Autodesk Inventor part; units mm, degrees
ref_plane "Work Plane1" through (-5.75, 2, 0) normal (0, 1, 0) x (1, 0, 0)
ref_plane "YZ Plane" through (0, 0, 0) normal (1, 0, 0) x (0, 1, 0)
ref_plane "XZ Plane" through (0, 0, 0) normal (0, 1, 0) x (-1, 0, 0)
sketch "Sketch1" plane through (0, 0, 0) normal (0, 0, 1) x (1, 0, 0)
  circle A0 centre (0, 0) radius 1
  circle A1 centre (0, 0) radius 1.75
  line L0 (-1.75, 0) -> (-1.75, -4)
  line L1 (-1.75, -4) -> (-5.75, -4)
  line L2 (-5.75, -4) -> (-5.75, -6)
  line L3 (-5.75, -6) -> (0, -6)
  line L4 (0, 0) -> (0, -6)
  line L5 (1.75, 0) -> (1.75, -4)
  line L6 (1.75, -4) -> (5.75, -4)
  line L7 (5.75, -4) -> (5.75, -6)
  line L8 (5.75, -6) -> (0, -6)
  dimension "d9" = 3.5
  dimension "d8" = 2
  dimension "d10" = 4
  dimension "d11" = 4
  dimension "d12" = 2
  dimension "d13" = 5.75
extrude "Extrusion1" add sketch "Sketch1" along normal blind 12
ref_plane "Work Plane1" through (-5.75, 2, 0) normal (0, 1, 0) x (1, 0, 0)
sketch "Sketch2" plane through (-5.75, 2, 0) normal (0, 1, 0) x (1, 0, 0)
  line L0 (7.5, 0) -> (7.5, -12)
  line L1 (4, 0) -> (7.5, 0)
  line L2 (4, 0) -> (4, -12)
  line L3 (4, -12) -> (7.5, -12)
  line L4 (6.75, -12) -> (4.75, -12) construction
  line L5 (5.75, -12) -> (5.75, 0) construction
  line L6 (7.5, -6) -> (4, -6) construction
  line L7 (4, 0) -> (4, -12) construction
  line L8 (7.5, -10.5) -> (4, -10.5)
  line L9 (4, -10.5) -> (4, -1.5)
  line L10 (4, -1.5) -> (7.5, -1.5)
  line L11 (7.5, -1.5) -> (7.5, -10.5)
  line L12 (7.5, -10.5) -> (4, -1.5) construction
  line L13 (4, -10.5) -> (7.5, -1.5) construction
  point P0 (5.75, -6)
  dimension "d17" = 9
extrude "Extrusion2" cut sketch "Sketch2" against normal blind 12 contours L0 L8 L2 L10
fillet "Fillet1" radius 2 4 edges at (1.75, -4, 0.75) (1.75, -4, 11.25) (-1.75, -4, 0.75) (-1.75, -4, 11.25)
fillet "Fillet2" radius 1 2 edges at (1.75, -4, 6) (-1.75, -4, 6)
sketch "Sketch3" plane through (-5.75, -4, 12) normal (0, 1, 0) x (1, 0, 0)
  line L0 (8.5, 1.5) -> (8.5, 10.5)
  line L1 (8.5, 1.5) -> (9.5, 1.5)
  line L2 (9.5, 0) -> (9.5, 1.5)
  line L3 (11.5, 0) -> (9.5, 0)
  line L4 (11.5, 12) -> (11.5, 0)
  line L5 (11.5, 12) -> (9.5, 12)
  line L6 (9.5, 10.5) -> (9.5, 12)
  line L7 (9.5, 10.5) -> (8.5, 10.5)
  line L8 (3, 10.5) -> (3, 1.5)
  line L9 (3, 10.5) -> (2, 10.5)
  line L10 (2, 12) -> (2, 10.5)
  line L11 (2, 12) -> (0, 12)
  line L12 (0, 12) -> (0, 0)
  line L13 (2, 0) -> (0, 0)
  line L14 (2, 1.5) -> (2, 0)
  line L15 (2, 1.5) -> (3, 1.5)
  line L16 (11.5, 12) -> (11.5, 0) construction
  line L17 (11.5, 6) -> (0, 6) construction
  line L18 (0, 12) -> (0, 0) construction
  circle A0 centre (9.5, 6) radius 1
  circle A1 centre (2, 6) radius 1
  point P0 (5.75, 12)
  dimension "d22" = 2
  dimension "d23" = 2
  dimension "d24" = 2
extrude "Extrusion3" cut sketch "Sketch3" against normal through all contours A0 | A1
properties part number "_3DPrint"
Work out the finished part from the listing and answer in its coordinate system (mm). A direction names the side the tool comes from. Round coordinates to 2 decimals unless told otherwise and drop trailing zeros. Order: outer loops, then holes, each group sorted by start corner. A loop starts at its lowest first (then second) coordinate and runs counter-clockwise, first axis right, second up. Notation, with made-up numbers: M 78,28 L 106,28 A25 cw 106,43 Z; hole C -36.75,81.5 d4. An arc over 180 degrees is marked long. One line per item, written item: value.
Q1. Flat-ended cylindrical pins translate along their axes: pin 1 (1.2 mm diameter, centred on x = -3.75, z = 6, fed in from -Y); pin 2 (1.5 mm diameter, centred on y = -1, z = 10.5, fed in from -X); pin 3 (1.6 mm diameter, centred on y = -1.5, z = 1, fed in from +X); pin 4 (0.9 mm diameter, centred on x = -4, z = 8.5, fed in from +Y). Find the tip coordinate at first contact, or state that the pin passes through.
Derived:
pin 1: through
pin 2: x = -1.75
pin 3: x = 1.77
pin 4: y = -4
Q2. Determine the mould class of faces 6 (the face through (-4.487, -4.986, 5.324)), 7 (the face through (-0.04, 1.75, 11.24)), 8 (the face through (0, 1, 11)) for opening direction Y: released by +Y, released by -Y, zero draft, split by the parting line, or undercut.
Derived:
face 6: zero draft
face 7: released by +Y
face 8: undercut
Q3. Find section B-B on x = 0. Write down the section's boundary in (y, z).
Derived:
outline: M -6,0 L -1,0 L -1,1.5 L -6,1.5 Z; M -6,10.5 L -1,10.5 L -1,12 L -6,12 Z; M 1,0 L 1.75,0 L 1.75,1.5 L 1,1.5 Z; M 1,10.5 L 1.75,10.5 L 1.75,12 L 1,12 Z
Q4. Find section C-C on y = -2.75. Write down the section's boundary in (x, z), then the cut area to 3 significant figures.
Derived:
outline: M -1.9,0 L 1.9,0 L 1.9,1.5 L -1.9,1.5 Z; M -1.9,10.5 L 1.9,10.5 L 1.9,12 L -1.9,12 Z
area: 11.4 mm²
Q5. Straight lines are drawn through the part: line 1 (X direction, y = -5.3, z = 6); line 2 (Z direction, x = 3.75, y = -4.5); line 3 (Y direction, x = 0, z = 0.5). For each, find the intervals that lie inside material, in ascending order.
Derived:
line 1: -5.75 to -4.75, -2.75 to -1.75, 1.75 to 2.75, 4.75 to 5.75
line 2: 0 to 5, 7 to 12
line 3: -6 to -1, 1 to 1.75
Q6. Find section A-A on z = 8.5. Write down the section's boundary in (x, y).
Derived:
outline: M -5.75,-6 L -1.75,-6 L -1.75,-5 A1 ccw -2.75,-4 L -5.75,-4 Z; M 1.75,-6 L 5.75,-6 L 5.75,-4 L 2.75,-4 A1 ccw 1.75,-5 Z
Q7. For faces 1 (the face through (5, -4, 6)), 2 (the face through (1.75, -1, 11)), 3 (the face through (-1.75, -1, 11)), 4 (the face through (-2.035, -4.301, 6.063)), 5 (the face through (-5, -4, 6)), determine the directions among +Z, -Z, +X, -X, +Y, -Y from which every point of the face is accessible in a straight line to the end or side of a thin tool.
Derived:
face 1: +X, +Y
face 2: +Z, -Z, +X, +Y
face 3: +Z, -Z, -X, +Y
face 4: +Y
face 5: -X, +Y
